from build123d import *

# Parameters (mm, degrees)
BOSS_EXTRUDE1_DEPTH = 6


with BuildPart() as part:
    # Sketch1 → Boss-Extrude1 (new body)
    with BuildSketch(Plane(origin=(0, 0, 0), x_dir=(0, 0, -1), z_dir=(1, 0, 0))):
        with BuildLine():
            Line((-95.25, 127.35), (-31.75, 0))
            Line((-31.75, 0), (-31.75, -6))
            Line((-31.75, -6), (-25.4, -6))
            Line((-25.4, -6), (-25.4, 0))
            Line((-25.4, 0), (-20.3835, 0))
            Line((-20.3835, 0), (-20.3835, 3.048))
            Line((-20.3835, 3.048), (-22.86, 3.048))
            Line((-22.86, 3.048), (-22.86, 6.096))
            Line((-22.86, 6.096), (-20.3835, 6.096))
            Line((-20.3835, 6.096), (-20.3835, 13.050000062))
            Line((-20.3835, 13.050000062), (-17.3355, 13.050000062))
            Line((-17.3355, 13.050000062), (-17.3355, 6.096))
            Line((-17.3355, 6.096), (-14.859, 6.096))
            Line((-14.859, 6.096), (-14.859, 3.048))
            Line((-14.859, 3.048), (-17.3355, 3.048))
            Line((-17.3355, 3.048), (-17.3355, 0))
            Line((-17.3355, 0), (-12.7, 0))
            Line((-12.7, 0), (-12.7, -6))
            Line((-12.7, -6), (-6.35, -6))
            Line((-6.35, -6), (-6.35, 0))
            Line((-6.35, 0), (-1.3335, 0))
            Line((-1.3335, 0), (-1.3335, 3.048))
            Line((-1.3335, 3.048), (-3.81, 3.048))
            Line((-3.81, 3.048), (-3.81, 6.096))
            Line((-3.81, 6.096), (-1.3335, 6.096))
            Line((-1.3335, 6.096), (-1.3335, 13.050000062))
            Line((-1.3335, 13.050000062), (1.7145, 13.050000062))
            Line((1.7145, 13.050000062), (1.7145, 6.096))
            Line((1.7145, 6.096), (4.191, 6.096))
            Line((4.191, 6.096), (4.191, 3.048))
            Line((4.191, 3.048), (1.7145, 3.048))
            Line((1.7145, 3.048), (1.7145, 0))
            Line((1.7145, 0), (6.35, 0))
            Line((6.35, 0), (6.35, -6))
            Line((6.35, -6), (12.7, -6))
            Line((12.7, -6), (12.7, 0))
            Line((12.7, 0), (17.7165, 0))
            Line((17.7165, 0), (17.7165, 3.048))
            Line((17.7165, 3.048), (15.24, 3.048))
            Line((15.24, 3.048), (15.24, 6.096))
            Line((15.24, 6.096), (17.7165, 6.096))
            Line((17.7165, 6.096), (17.7165, 13.050000062))
            Line((17.7165, 13.050000062), (20.7645, 13.050000062))
            Line((20.7645, 13.050000062), (20.7645, 6.096))
            Line((20.7645, 6.096), (23.241, 6.096))
            Line((23.241, 6.096), (23.241, 3.048))
            Line((23.241, 3.048), (20.7645, 3.048))
            Line((20.7645, 3.048), (20.7645, 0))
            Line((20.7645, 0), (25.4, 0))
            Line((25.4, 0), (25.4, -6))
            Line((25.4, -6), (31.75, -6))
            Line((31.75, -6), (31.75, 0))
            Line((31.75, 0), (31.75, 6.135772776))
            ThreePointArc((31.75, 6.135772776), (30.94204324, 12.491196387), (28.569574073, 18.442296576))
            Line((28.569574073, 18.442296576), (-31.75, 127.35))
            Line((-31.75, 127.35), (-37.465, 127.35))
            Line((-37.465, 127.35), (-37.465, 133.35))
            Line((-37.465, 133.35), (-46.355, 133.35))
            Line((-46.355, 133.35), (-46.355, 127.35))
            Line((-46.355, 127.35), (-51.3715, 127.35))
            Line((-51.3715, 127.35), (-51.3715, 124.302))
            Line((-51.3715, 124.302), (-48.895, 124.302))
            Line((-48.895, 124.302), (-48.895, 121.254))
            Line((-48.895, 121.254), (-51.3715, 121.254))
            Line((-51.3715, 121.254), (-51.3715, 114.299999938))
            Line((-51.3715, 114.299999938), (-54.4195, 114.299999938))
            Line((-54.4195, 114.299999938), (-54.4195, 121.254))
            Line((-54.4195, 121.254), (-56.896, 121.254))
            Line((-56.896, 121.254), (-56.896, 124.302))
            Line((-56.896, 124.302), (-54.4195, 124.302))
            Line((-54.4195, 124.302), (-54.4195, 127.35))
            Line((-54.4195, 127.35), (-59.055, 127.35))
            Line((-59.055, 127.35), (-59.055, 133.35))
            Line((-59.055, 133.35), (-67.945, 133.35))
            Line((-67.945, 133.35), (-67.945, 127.35))
            Line((-67.945, 127.35), (-72.9615, 127.35))
            Line((-72.9615, 127.35), (-72.9615, 124.302))
            Line((-72.9615, 124.302), (-70.485, 124.302))
            Line((-70.485, 124.302), (-70.485, 121.254))
            Line((-70.485, 121.254), (-72.9615, 121.254))
            Line((-72.9615, 121.254), (-72.9615, 114.299999938))
            Line((-72.9615, 114.299999938), (-76.0095, 114.299999938))
            Line((-76.0095, 114.299999938), (-76.0095, 121.254))
            Line((-76.0095, 121.254), (-78.486, 121.254))
            Line((-78.486, 121.254), (-78.486, 124.302))
            Line((-78.486, 124.302), (-76.0095, 124.302))
            Line((-76.0095, 124.302), (-76.0095, 127.35))
            Line((-76.0095, 127.35), (-80.645, 127.35))
            Line((-80.645, 127.35), (-80.645, 133.35))
            Line((-80.645, 133.35), (-95.25, 133.35))
            Line((-95.25, 133.35), (-95.25, 127.35))
        make_face()
    extrude(amount=BOSS_EXTRUDE1_DEPTH)


solid = part.part
CAD build for the part. Positions are in the model's coordinates, mm. A direction names the side the tool comes from. Give positions to 0.01 mm unless a question says otherwise; leave off trailing zeros. Loops run counter-clockwise (first coordinate to the right, second up) from the corner with the lowest first, then second, coordinate; pieces in that order, holes last. Notation, with made-up numbers: M 53,20.25 L 59,20.25 A25 cw 59,42.25 Z; hole C 61,73.25 d2. An arc over 180 degrees is marked long. Write each question's results on one line, items separated by ' | '.
Q1. Band-saw the part on C-C on y = 31. Write the cut outline in (x, z), and give its area (3 significant figures).
Geometry check:
outline: M 0,-21.61 L 6,-21.61 L 6,47.21 L 0,47.21 Z | area: 413 mm²
Q2. Probe probe 1 along Z at (x, y) = (4.9, 10); probe 2 along Y at (x, z) = (0.7, 22.5); probe 3 along Y at (x, z) = (3.3, 16). List the from-to ranges inside material, lowest first.
Geometry check:
probe 1: z = -31.45 to -20.76, -17.72 to -1.71, 1.33 to 17.34, 20.38 to 36.74 | probe 2: y = 0 to 3.05, 6.1 to 110.65 | probe 3: y = 0 to 3.05, 6.1 to 98.91
Q3. Which spindle directions (+Z, -Z, +X, -X, +Y, -Y) get a long thin tool onto all of the face, cutting with end or side? Do faces 4 (the face through (3, 5, 22.86)), 5 (the face through (3, 0, -23)), 6 (the face through (3, 130, 67.945)). Say none if no direction does.
Geometry check:
face 4: +X, -X | face 5: +X, -X, -Y | face 6: +X, -X, +Y
Q4. Flat gauge pins, fed straight in: P1, Ø1.5, axis at x = 3, z = 24, coming from the -Y side; P2, Ø1.8, axis at x = 2, y = -4.5, coming from the +Z side; P3, Ø1.2, axis at x = 3, z = -16, coming from the +Y side. Where does each tip first touch, or does it go through?
Geometry check:
P1: stops at y = 0 | P2: stops at z = 31.75 | P3: stops at y = 42.22
Q5. Mould opens along Z. For faces 1 (the face through (3, 126, 54.42)), 2 (the face through (2.958, 12.404, -30.964)), 3 (the face through (3, -6, -9)) say: pulls with the +Z half, pulls with the -Z half, needs draft (parallel to the pull), parting line crosses it, or undercut.
Geometry check:
face 1: undercut | face 2: pulls with the -Z half | face 3: needs draft
Q6. Band-saw the part on A-A on y = 119. Write the cut outline in (x, z), and give its area (3 significant figures).
Geometry check:
outline: M 0,27.13 L 6,27.13 L 6,51.37 L 0,51.37 Z; M 0,54.42 L 6,54.42 L 6,72.96 L 0,72.96 Z; M 0,76.01 L 6,76.01 L 6,91.09 L 0,91.09 Z | area: 347 mm²
Q7. Band-saw the part on B-B on y = 82.5. Write the cut outline in (x, z).
Geometry check:
outline: M 0,6.91 L 6,6.91 L 6,72.89 L 0,72.89 Z
